Geometry check sheet. Reference: the model listing, model coordinates, mm. A direction names the side the tool comes from. Coordinates: 2 decimals unless noted, no trailing zeros. Write each loop counter-clockwise with the first axis right and the second up, starting at its lowest first coordinate (ties: lowest second). Pieces come first, ordered by that corner, then holes. Notation, with made-up numbers: (-25, 27.5) -> (-3, 27.5) arc R15 cw to (-3, 49.5) -> close; hole circle Ø4 at (12.5, 21). An arc over 180 degrees is marked (long way). Answer as CSV lines item,"result".
```python
from build123d import *

# Parameters (mm, degrees)
SKETCH4_R        = 20
SKETCH4_R_2      = 5.5
SKETCH4_R_3      = 4.75
LIDBASE_DEPTH    = 7.5
SKETCH5_R        = 18.25
LIDGROOVES_DEPTH = 4


with BuildPart() as part:
    # Sketch4 → LidBase (new body)
    with BuildSketch(Plane(origin=(0, 0, 0), x_dir=(1, 0, 0), z_dir=(0, 1, 0))):
        Circle(SKETCH4_R)
        Circle(SKETCH4_R_2, mode=Mode.SUBTRACT)
        with Locations((0, 11.125)):
            Circle(SKETCH4_R_3, mode=Mode.SUBTRACT)
        with Locations((0, -11.125)):
            Circle(SKETCH4_R_3, mode=Mode.SUBTRACT)
    extrude(amount=LIDBASE_DEPTH)

    # Sketch5 → LidGrooves (cut)
    with BuildSketch(Plane(origin=(0, 7.5, 0), x_dir=(1, 0, 0), z_dir=(0, 1, 0))):
        Circle(SKETCH5_R)
    extrude(amount=-LIDGROOVES_DEPTH, mode=Mode.SUBTRACT)


solid = part.part
```
Item 1: Thickness scan on probe 1 along Z at (x, y) = (0, 1.25) (3 decimals); probe 2 along Z at (x, y) = (-2, 0.5); probe 3 along X at (y, z) = (6.65, 0). Record the ranges inside material, lowest first.
Responses:
probe 1,"z = -20 to -15.875, -6.375 to -5.5, 5.5 to 6.375, 15.875 to 20"
probe 2,"z = -19.9 to -15.43, -6.82 to -5.12, 5.12 to 6.82, 15.43 to 19.9"
probe 3,"x = -20 to -18.25, 18.25 to 20"
Item 2: Depth check by flat-ended pin: pin 1 Ø2 at (x, y) = (3.5, 5) entering from -Z; pin 2 Ø3 at (y, z) = (1, -0.5) entering from +X; pin 3 Ø2 at (x, y) = (15.5, 1.5) entering from +Z (3 decimals); pin 4 Ø1.5 at (y, z) = (5, 7.5) entering from +X. Enter the tip coordinate at first touch or a pass-through.
Responses:
pin 1,"stops at z = -19.84"
pin 2,"stops at x = 20"
pin 3,"stops at z = 13.775"
pin 4,"stops at x = 18.83"
Item 3: Set-up check for faces 1 (the cylindrical face through (-3.956, 5.528, 17.816)), 2 (the cylindrical face through (-1.19, 1.73, 5.37)): record each of +Z, -Z, +X, -X, +Y, -Y from which the full face is reachable in a straight line by a thin tool's end or side.
Responses:
face 1,"+Y"
face 2,"+Y, -Y"
Item 4: Release check for a two-part mould opening along Z. For faces 3 (the cylindrical face through (-1.03, 1.73, -6.49)), 4 (the cylindrical face through (-4.336, 3.698, 19.524)), 5 (the flat face through (4, 0, 4)) record: +Z half, -Z half, draft (parallel to the pull), parting line (faces both ways), or undercut.
Responses:
face 3,"undercut"
face 4,"parting line"
face 5,"draft"
Item 5: Cross-section at C-C, the plane y = 6.5. Record the cut outline in (x, z).
Responses:
outline,"circle Ø40 at (0, 0); hole circle Ø36.5 at (0, 0)"
Item 6: Cross-section at B-B, the plane z = 0. Record the cut outline in (x, y).
Responses:
outline,"(-20, 0) -> (-5.5, 0) -> (-5.5, 3.5) -> (-18.25, 3.5) -> (-18.25, 7.5) -> (-20, 7.5) -> close; (5.5, 0) -> (20, 0) -> (20, 7.5) -> (18.25, 7.5) -> (18.25, 3.5) -> (5.5, 3.5) -> close"
Item 7: Cross-section at A-A, the plane x = 0. Record the cut outline in (y, z) (3 decimals), plus the area to 3 significant figures.
Responses:
outline,"(0, -20) -> (7.5, -20) -> (7.5, -18.25) -> (3.5, -18.25) -> (3.5, -15.875) -> (0, -15.875) -> close; (0, -6.375) -> (3.5, -6.375) -> (3.5, -5.5) -> (0, -5.5) -> close; (0, 5.5) -> (3.5, 5.5) -> (3.5, 6.375) -> (0, 6.375) -> close; (0, 15.875) -> (3.5, 15.875) -> (3.5, 18.25) -> (7.5, 18.25) -> (7.5, 20) -> (0, 20) -> close"
area,"49.0 mm2"
Item 8: Cross-section at D-D, the plane x = -14.5. Record the cut outline in (y, z).
Responses:
outline,"(0, -13.77) -> (7.5, -13.77) -> (7.5, -11.08) -> (3.5, -11.08) -> (3.5, 11.08) -> (7.5, 11.08) -> (7.5, 13.77) -> (0, 13.77) -> close"
